from build123d import *

# Parameters (mm, degrees)
SKIZZE1_W                       = 61
SKIZZE1_H                       = 96.5
SKIZZE1_R                       = 0.5
AUFSATZ_LINEAR_AUSTRAGEN1_DEPTH = 1.6


with BuildPart() as part:
    # Skizze1 → Aufsatz-Linear austragen1 (new body)
    with BuildSketch(Plane.XY):
        with Locations((0, -11.75)):
            Rectangle(SKIZZE1_W, SKIZZE1_H)
        with Locations((0, 30.5)):
            Circle(SKIZZE1_R, mode=Mode.SUBTRACT)
        with Locations((-24.5, -28)):
            Circle(SKIZZE1_R, mode=Mode.SUBTRACT)
        with Locations((24.5, -28)):
            Circle(SKIZZE1_R, mode=Mode.SUBTRACT)
        with BuildLine():
            Line((-22.231560855, -53), (-15.190457531, -53))
            ThreePointArc((-15.190457531, -53), (-9.397914174, -48.720244698), (-2.5, -46.649340538))
            Line((-2.5, -46.649340538), (-2.5, -45))
            ThreePointArc((-2.5, -45), (-2.207106781, -44.292893219), (-1.5, -44))
            Line((-1.5, -44), (1.5, -44))
            ThreePointArc((1.5, -44), (2.207106781, -44.292893219), (2.5, -45))
            Line((2.5, -45), (2.5, -46.649340538))
            ThreePointArc((2.5, -46.649340538), (9.397914174, -48.720244698), (15.190457531, -53))
            Line((15.190457531, -53), (22.231560855, -53))
            ThreePointArc((22.231560855, -53), (23.135640421, -41.41122194), (23.493493996, -29.792741935))
            ThreePointArc((23.493493996, -29.792741935), (24.50072572, -28.80002634), (25.493441316, -29.807258065))
            ThreePointArc((25.493441316, -29.807258065), (25.125648184, -41.648701954), (24.195027533, -53.459248528))
            ThreePointArc((24.195027533, -53.459248528), (23.637637029, -54.557859223), (22.487793054, -55))
            Line((22.487793054, -55), (15.068542623, -55))
            ThreePointArc((15.068542623, -55), (14.388773301, -54.859637633), (13.820194306, -54.461509699))
            ThreePointArc((13.820194306, -54.461509699), (0, -48.5), (-13.820194306, -54.461509699))
            ThreePointArc((-13.820194306, -54.461509699), (-14.388773301, -54.859637633), (-15.068542623, -55))
            Line((-15.068542623, -55), (-22.487793054, -55))
            ThreePointArc((-22.487793054, -55), (-23.637637029, -54.557859223), (-24.195027533, -53.459248528))
            ThreePointArc((-24.195027533, -53.459248528), (-25.125648184, -41.648701954), (-25.493441316, -29.807258065))
            ThreePointArc((-25.493441316, -29.807258065), (-24.50072572, -28.80002634), (-23.493493996, -29.792741935))
            ThreePointArc((-23.493493996, -29.792741935), (-23.135640421, -41.41122194), (-22.231560855, -53))
        make_face(mode=Mode.SUBTRACT)
        with BuildLine():
            Line((-19, 5), (-21.285620493, 5))
            ThreePointArc((-21.285620493, 5), (-19.763470557, 14.80051276), (-17.849098235, 24.532016724))
            ThreePointArc((-17.849098235, 24.532016724), (-17.173923296, 25.871247857), (-15.934850806, 26.716292583))
            ThreePointArc((-15.934850806, 26.716292583), (-8.95491897, 28.639022814), (-1.7625, 29.466941499))
            ThreePointArc((-1.7625, 29.466941499), (-0.800703372, 30.503738126), (-1.8375, 31.465534754))
            ThreePointArc((-1.8375, 31.465534754), (-9.335979351, 30.602385487), (-16.612929564, 28.597836948))
            ThreePointArc((-16.612929564, 28.597836948), (-18.67805038, 27.189429071), (-19.803341946, 24.957377183))
            ThreePointArc((-19.803341946, 24.957377183), (-21.761478169, 14.986129467), (-23.311141633, 4.943290145))
            ThreePointArc((-23.311141633, 4.943290145), (-22.901341819, 3.585796991), (-21.609999326, 3))
            Line((-21.609999326, 3), (-19, 3))
            ThreePointArc((-19, 3), (-16, 0), (-19, -3))
            Line((-19, -3), (-22.685152712, -3))
            ThreePointArc((-22.685152712, -3), (-23.84016455, -3.446823778), (-24.39375693, -4.554632116))
            ThreePointArc((-24.39375693, -4.554632116), (-25.179058013, -15.361720617), (-25.493441316, -26.192741935))
            ThreePointArc((-25.493441316, -26.192741935), (-24.50072572, -27.19997366), (-23.493493996, -26.207258065))
            ThreePointArc((-23.493493996, -26.207258065), (-23.188154433, -15.592161252), (-22.426818383, -5))
            Line((-22.426818383, -5), (-19, -5))
            ThreePointArc((-19, -5), (-14, 0), (-19, 5))
        make_face(mode=Mode.SUBTRACT)
        with BuildLine():
            Line((19, 5), (21.285620493, 5))
            ThreePointArc((21.285620493, 5), (19.763470557, 14.80051276), (17.849098235, 24.532016724))
            ThreePointArc((17.849098235, 24.532016724), (17.173923296, 25.871247857), (15.934850806, 26.716292583))
            ThreePointArc((15.934850806, 26.716292583), (8.95491897, 28.639022814), (1.7625, 29.466941499))
            ThreePointArc((1.7625, 29.466941499), (0.800703372, 30.503738126), (1.8375, 31.465534754))
            ThreePointArc((1.8375, 31.465534754), (9.335979351, 30.602385487), (16.612929564, 28.597836948))
            ThreePointArc((16.612929564, 28.597836948), (18.67805038, 27.189429071), (19.803341946, 24.957377183))
            ThreePointArc((19.803341946, 24.957377183), (21.761478169, 14.986129467), (23.311141633, 4.943290145))
            ThreePointArc((23.311141633, 4.943290145), (22.901341819, 3.585796991), (21.609999326, 3))
            Line((21.609999326, 3), (19, 3))
            ThreePointArc((19, 3), (16, 0), (19, -3))
            Line((19, -3), (22.685152712, -3))
            ThreePointArc((22.685152712, -3), (23.84016455, -3.446823778), (24.39375693, -4.554632116))
            ThreePointArc((24.39375693, -4.554632116), (25.179058013, -15.361720617), (25.493441316, -26.192741935))
            ThreePointArc((25.493441316, -26.192741935), (24.50072572, -27.19997366), (23.493493996, -26.207258065))
            ThreePointArc((23.493493996, -26.207258065), (23.188154433, -15.592161252), (22.426818383, -5))
            Line((22.426818383, -5), (19, -5))
            ThreePointArc((19, -5), (14, 0), (19, 5))
        make_face(mode=Mode.SUBTRACT)
    extrude(amount=AUFSATZ_LINEAR_AUSTRAGEN1_DEPTH)


solid = part.part
Geometry check sheet. Reference: the model listing, model coordinates, mm. A direction names the side the tool comes from. Round coordinates to 2 decimals unless told otherwise and drop trailing zeros. Write each loop counter-clockwise with the first axis right and the second up, starting at its lowest first coordinate (ties: lowest second). Pieces come first, ordered by that corner, then holes.
Item 1: Mould release check, pull along X, two halves, no side actions. Record for faces 1 (the face through (16, 0, 1)), 2 (the face through (0, -11, 1.6)): +X half, -X half, draft (parallel to the pull), parting line (faces both ways), or undercut.
Determined:
face 1: undercut
face 2: draft
Item 2: Section check D-D (z = 1.15). Give the number of separate pieces and of enclosed holes in the cut face, plus the area to 3 significant figures.
Determined:
separate pieces: 1
enclosed holes: 6
area: 5,340 mm2
Item 3: Material ranges on line 1 along X through (y, z) = (-34, 0.8); line 2 along X through (y, z) = (-37, 1.1); line 3 along Y through (x, z) = (10, 0.3), recorded low to high.
Determined:
line 1: x = -30.5 to -25.43, -23.43 to 23.43, 25.43 to 30.5
line 2: x = -30.5 to -25.34, -23.34 to 23.34, 25.34 to 30.5
line 3: y = -60 to -51.34, -49.03 to 28.42, 30.47 to 36.5
Item 4: Access from +Z, -Z, +X, -X, +Y, -Y to the whole of each face (thin tool, end or side, straight path). Record for faces 3 (the face through (17.188, 25.855, 0.789)), 4 (the face through (0, -11, 0)).
Determined:
face 3: +Z, -Z
face 4: -Z, +X, -X, +Y, -Y
Item 5: Section check B-B (y = -50.5). Record the boundary of the cut face in (x, z), plus the area to 3 significant figures.
Determined:
outline: (-30.5, 0) - (-24.48, 0) - (-24.48, 1.6) - (-30.5, 1.6) - close; (-22.47, 0) - (-12.33, 0) - (-12.33, 1.6) - (-22.47, 1.6) - close; (-8.49, 0) - (8.49, 0) - (8.49, 1.6) - (-8.49, 1.6) - close; (12.33, 0) - (22.47, 0) - (22.47, 1.6) - (12.33, 1.6) - close; (24.48, 0) - (30.5, 0) - (30.5, 1.6) - (24.48, 1.6) - close
area: 78.9 mm2
Item 6: Section check C-C (x = 5.5). Record the boundary of the cut face in (y, z).
Determined:
outline: (-60, 0) - (-49.31, 0) - (-49.31, 1.6) - (-60, 1.6) - close; (-47.23, 0) - (29.18, 0) - (29.18, 1.6) - (-47.23, 1.6) - close; (31.19, 0) - (36.5, 0) - (36.5, 1.6) - (31.19, 1.6) - close
Item 7: Section check A-A (y = 0). Record the boundary of the cut face in (x, z).
Determined:
outline: (-30.5, 0) - (-16, 0) - (-16, 1.6) - (-30.5, 1.6) - close; (-14, 0) - (14, 0) - (14, 1.6) - (-14, 1.6) - close; (16, 0) - (30.5, 0) - (30.5, 1.6) - (16, 1.6) - close
